Geometry: final body of the model. Coordinates: model frame, mm. Face numbers are marked on the shaded views. A direction names the side the tool comes from. Give positions to 0.01 mm unless a question says otherwise; leave off trailing zeros. Write each loop counter-clockwise with the first axis right and the second up, starting at its lowest first coordinate (ties: lowest second). Pieces come first, ordered by that corner, then holes. Notation, with made-up numbers: (62, 38.5) -> (101, 38.5) arc R22 cw to (101, 54.5) -> close; hole circle Ø10 at (77.5, -15.75). An arc over 180 degrees is marked (long way). Answer in a Markdown table with one row per item. Add a question column.
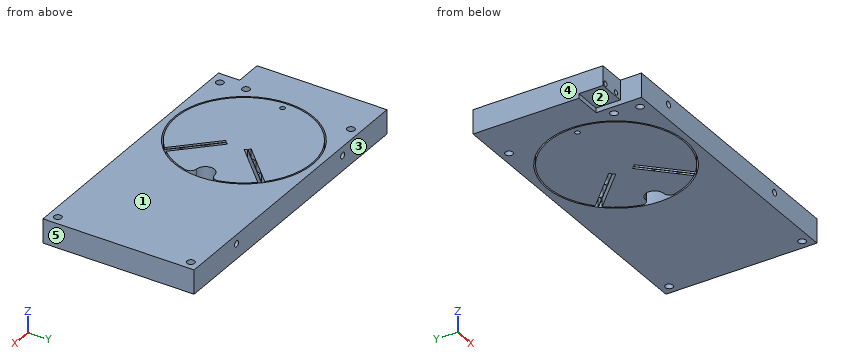
Autodesk Inventor part; units mm, degrees
ref_plane "YZ Plane" through (0, 0, 0) normal (1, 0, 0) x (0, 1, 0)
ref_plane "XZ Plane" through (0, 0, 0) normal (0, 1, 0) x (-1, 0, 0)
ref_plane "XY Plane" through (0, 0, 0) normal (0, 0, 1) x (1, 0, 0)
sketch "Sketch1" plane through (0, 0, 0) normal (0, 0, 1) x (1, 0, 0)
  line L0 (0, 0) -> (100, 0)
  line L1 (100, 0) -> (100, 50)
  line L2 (100, 50) -> (0, 50)
  line L3 (0, 50) -> (0, 0)
  circle A0 centre (95, 45) radius 1.75
  circle A1 centre (95, 5) radius 1.75
  circle A2 centre (15, 45) radius 1.75
  circle A3 centre (15, 5) radius 1.75
  dimension "d0" = 50
  dimension "d1" = 100
  dimension "d2" = 5
  dimension "d3" = 5
  dimension "d4" = 5
  dimension "d5" = 5
  dimension "d6" = 5
  dimension "d7" = 15
  dimension "d8" = 15
  dimension "d9" = 5
  dimension "d10" = 3.5
  dimension "d11" = 3.5
  dimension "d12" = 3.5
  dimension "d13" = 3.5
extrude "Extrusion1" add sketch "Sketch1" along normal blind 8 contours L3 L2 L1 L0 | A0 | A1 | A2 | A3
sketch "Sketch4" plane through (0, 0, 8) normal (0, 0, 1) x (1, 0, 0)
  circle A0 centre (15, 25) radius 0.8
  circle A1 centre (55, 25) radius 3
  line L0 (0, 50) -> (0, 0)
  line L1 (35, 25) -> (52.9141, 42.9141)
  line L2 (35, 25) -> (41.4896, 25)
  line L3 (35, 25) -> (55.1987, 4.8013)
  circle A2 centre (35, 25) radius 23
  line L4 (0, 0) -> (100, 0)
  circle A3 centre (35, 25) radius 5
  line L5 (38.5, 28.5707) -> (51.2281, 41.2988)
  line L6 (37.757, 29.1712) -> (50.1871, 41.6013)
  line L7 (38.5707, 28.5) -> (51.2988, 41.2281)
  line L8 (51.6013, 40.1871) -> (39.1712, 27.757)
  line L9 (38.5707, 21.5) -> (51.2988, 8.7719)
  line L10 (38.5, 21.4293) -> (51.2281, 8.7012)
  line L11 (37.757, 20.8288) -> (50.1871, 8.3987)
  line L12 (39.1712, 22.243) -> (51.6013, 9.8129)
  arc A4 (51.6013, 9.8129) -> (50.1871, 8.3987) centre (35, 25) ccw
  circle A5 centre (41.2925, 32.7067) radius 0.95
  circle A6 centre (42.7067, 34.121) radius 0.95
  circle A7 centre (46.2423, 37.6565) radius 0.95
  circle A8 centre (47.6565, 39.0707) radius 0.95
  circle A9 centre (42.7067, 18.7075) radius 0.95
  circle A10 centre (44.121, 17.2933) radius 0.95
  circle A11 centre (47.6565, 13.7577) radius 0.95
  circle A12 centre (49.0707, 12.3435) radius 0.95
  point P0 (0, 15)
  point P1 (7, 0)
  point P2 (57.4312, 26.7576)
  point P3 (57.4312, 23.2424)
  point P4 (58, 25)
  point P5 (50.9452, 40.8745)
  point P6 (50.8745, 40.9452)
  point P7 (41.9643, 32.035)
  point P8 (41.9643, 33.3785)
  point P9 (42.035, 33.4492)
  point P10 (43.3785, 33.4492)
  point P11 (46.914, 36.9847)
  point P12 (46.914, 38.3282)
  point P13 (48.3282, 38.399)
  point P14 (46.9847, 38.399)
  point P15 (42.035, 18.0357)
  point P16 (43.3785, 18.0357)
  point P17 (43.4492, 17.965)
  point P18 (43.4492, 16.6215)
  point P19 (46.9847, 13.086)
  point P20 (48.3282, 13.086)
  point P21 (48.399, 13.0153)
  point P22 (48.399, 11.6718)
  dimension "d34" = 10
  dimension "d22" = 15
  dimension "d23" = 40
  dimension "d24" = 20
  dimension "d26" = 1.6
  dimension "d27" = 6
  dimension "d28" = 45
  dimension "d29" = 45
  dimension "d30" = 46
  dimension "d31" = 25
  dimension "d32" = 25
  dimension "d33" = 25
  dimension "d35" = 1
  dimension "d36" = 1
  dimension "d37" = 0.1
  dimension "d38" = 0.05
  dimension "d39" = 0.1
  dimension "d40" = 0.05
  dimension "d41" = 1
  dimension "d42" = 1
  dimension "d79" = 5
  dimension "d80" = 2
  dimension "d81" = 5
  dimension "d82" = 2
  dimension "d83" = 5
  dimension "d84" = 2
  dimension "d85" = 5
  dimension "d86" = 2
extrude "Extrusion4" cut sketch "Sketch4" against normal blind 8 contours A0 | A1 A4 | A2 L9 A12 L12 A4 A1 | A1 A4 L7 A2 | A4 A1 | L8 A3 L7 A4 | A12 L12 | L5 A4 L11 A3 L10 A2 | L9 A10 L12 A11 | A11 L12 | L5 A8 L6 A4 | A3 L12 A9 L9 | A10 L12 | A3 L6 A5 L5 | A8 L6 | A9 L12 | A5 L6 | L5 A6 L6 A7 | A7 L6 | A6 L6 picked at (49.0352, 12.0288) picked at (47.3576, 13.4145) picked at (44.1564, 16.9786) picked at (47.9671, 39.0089) picked at (42.6021, 18.4086) picked at (41.6092, 32.7067) picked at (46.2068, 37.3418) picked at (43.0173, 33.7349)
fillet "Fillet2" radius 2 2 edges at (57.4312, 26.7576, 4) (57.4312, 23.2424, 4)
sketch "Sketch5" plane through (0, 0, 0) normal (-1, 0, 0) x (0, 0, 1)
  line L0 (0, 0) -> (1.5, 0)
  line L1 (1.5, 0) -> (1.5, 15)
  line L2 (1.5, 15) -> (0, 15)
  line L3 (0, 15) -> (0, 0)
  line L4 (8, 0) -> (8, 50)
  line L5 (8, 0) -> (1.5, 0)
  line L6 (1.5, 0) -> (1.5, 7)
  line L7 (1.5, 7) -> (8, 7)
  line L8 (8, 7) -> (8, 0)
  dimension "d47" = 15
  dimension "d48" = 1.5
  dimension "d51" = 7
extrude "Extrusion5" cut sketch "Sketch5" against normal blind 9
sketch "Sketch6" plane through (0, 7, 1.5) normal (0, -1, 0) x (1, 0, 0)
  circle A0 centre (6.75, 1.2764) radius 1.1
  circle A1 centre (1.25, 1.2764) radius 1.1
  circle A2 centre (6.75, 1.2764) radius 0.8
  circle A3 centre (1.25, 1.2764) radius 0.8
  point P0 (0, -1.5)
  dimension "d52" = 1.6
  dimension "d53" = 1.6
extrude "Extrusion6" cut sketch "Sketch6" against normal blind 8 contours A2 | A3
sketch "Sketch7" plane through (0, 0, 8) normal (0, 0, 1) x (1, 0, 0)
  circle A0 centre (97, 3) radius 1.7
  circle A1 centre (97, 47) radius 1.7
  circle A2 centre (12, 11) radius 1.7
  circle A3 centre (21.5, 47.5) radius 1.7
  circle A4 centre (97, 3) radius 1.25
  circle A5 centre (97, 47) radius 1.25
  circle A6 centre (13, 3) radius 1.25
  circle A7 centre (12, 11) radius 1.25
  circle A8 centre (21.5, 47.5) radius 1.25
  circle A9 centre (14, 47) radius 1.7
  circle A10 centre (14, 47) radius 1.25
  line L0 (9, 0) -> (100, 0)
  line L1 (9, 0) -> (9, 15)
  point P0 (0, 0)
  dimension "d56" = 2.5
  dimension "d57" = 2.5
  dimension "d58" = 2.5
  dimension "d59" = 2.5
  dimension "d60" = 2.5
  dimension "d63" = 2.5
  dimension "d64" = 3
  dimension "d65" = 4
extrude "Extrusion7" cut sketch "Sketch7" against normal blind 8 contours A4 | A5 | A6 | A7 | A10
sketch "Sketch8" plane through (0, 50, 0) normal (0, 1, 0) x (1, 0, 0)
  circle A0 centre (23, -5) radius 1.375
  circle A1 centre (78, -5) radius 1.375
  circle A2 centre (23, -5) radius 1.025
  circle A3 centre (78, -5) radius 1.025
  line L0 (0, 0) -> (0, -8)
  dimension "d68" = 2.05
  dimension "d69" = 2.05
  dimension "d74" = 23
  dimension "d75" = 23
  dimension "d76" = 55
extrude "Extrusion8" cut sketch "Sketch8" against normal blind 8 contours A2 | A3
sketch "Sketch9" plane through (100, 0, 0) normal (0, -1, 0) x (1, 0, 0)
  circle A0 centre (-77, 5) radius 1.375
  circle A1 centre (-22, 5) radius 1.375
  circle A2 centre (-77, 5) radius 1.025
  circle A3 centre (-22, 5) radius 1.025
  line L0 (-100, 1.5) -> (-100, 8)
  point P0 (-100, 0)
  dimension "d70" = 2.05
  dimension "d71" = 2.05
  dimension "d77" = 23
  dimension "d78" = 55
extrude "Extrusion9" cut sketch "Sketch9" against normal blind 8 contours A2 | A3
equation "\"d4\" = d3"
equation "\"d5\" = d2"
equation "\"d6\" = d3"
equation "\"d9\" = d4"
equation "\"d10\" = d11"
equation "\"d12\" = d11"
equation "\"d13\" = d11"
equation "\"d24\" = 0.5 * d23"
equation "\"d37\" = BladeThicknessRCC"
equation "\"d38\" = 0.5 * d37"
equation "\"d39\" = BladeThicknessRCC"
equation "\"d40\" = 0.5 * BladeThicknessRCC"
equation "\"d59\" = d58"
equation "\"d60\" = d59"
equation "\"d75\" = d74"
equation "\"bladeThicknessTablePushing\" = 0.1"
equation "\"bladeThicknessTable\" = 0.1"
equation "\"bladeThicknessForceConverter\" = 0.2"
equation "\"bladeThicknessWheelAnchor\" = 0.1"
equation "\"safetyPlay\" = 0.1"
equation "\"OffsetMotorSpring\" = -1"
equation "\"BladeThicknessRCC\" = 0.1"
equation "\"bladeThicknessZeroConverter\" = 0.1"
equation "\"rangeXProbeMin\" = -0.6"
equation "\"thicknessWheelPlate\" = 8"
equation "\"rangeXProbeMax\" = 0.6"
equation "\"BladeLengthRCC\" = 18"
equation "\"bladeLengthTable\" = 18"
equation "\"bladeLengthWheelAnchor\" = 7.5"
equation "\"RCCdeadCenter\" = 5"
equation "\"bladeLengthZeroConverter\" = 11.98"
equation "\"bladeLengthTablePushing\" = 12"
equation "\"bladeLengthForceConverter\" = 12.125"
equation "\"thicknessConverterPlate\" = 4"
properties part number "RoueV3partA"
Q1. Section B-B on x = 46. Return loops of the section in (y, z), and give its area (3 significant figures).
Q2. Pull-direction query (X, two-part tool) for the marked faces 3, 4 and 5; classes: +X half, -X half, draft (parallel to the pull), parting line (faces both ways), or undercut.
Q3. Contact query for flat-ended pins moving along their axis: pin 1 Ø2.5 at (x, z) = (23, 5) entering from -Y; pin 2 Ø1.3 at (x, z) = (6.5, 2.5) entering from -Y; pin 3 Ø1.8 at (x, z) = (78, 5) entering from -Y; pin 4 Ø4 at (x, y) = (6, 12) entering from -Z. Output: stop coordinate, or through.
Q4. Line query: probe 1 along Z at (x, y) = (78, 44) (3 decimals); probe 2 along X at (y, z) = (23.5, 6.25); probe 3 along X at (y, z) = (12, 7). Output: solid intervals per line, ascending. Write a range as from..to.
Q5. Access query for the marked faces 1 and 2. Directions: +Z, -Z, +X, -X, +Y, -Y. A direction counts if a zero-diameter tool reaches every point of the face in a straight line with its end or side. Return the directions, or none.
Q6. Section A-A on x = 35. Return loops of the section in (y, z), and give its area (3 significant figures).
Checks:
| question | item | result |
|---|---|---|
| 1 | outline | (0, 0) -> (4.8, 0) -> (4.8, 8) -> (0, 8) -> close; (5.37, 0) -> (12.59, 0) -> (12.59, 8) -> (5.37, 8) -> close; (13.93, 0) -> (14.07, 0) -> (14.07, 8) -> (13.93, 8) -> close; (15.41, 0) -> (34.59, 0) -> (34.59, 8) -> (15.41, 8) -> close; (35.93, 0) -> (36.07, 0) -> (36.07, 8) -> (35.93, 8) -> close; (37.41, 0) -> (44.63, 0) -> (44.63, 8) -> (37.41, 8) -> close; (45.2, 0) -> (50, 0) -> (50, 8) -> (45.2, 8) -> close |
| 1 | area | 348 mm^2 |
| 2 | face 3 | draft |
| 2 | face 4 | -X half |
| 2 | face 5 | +X half |
| 3 | pin 1 | y = 0 |
| 3 | pin 2 | y = 7 |
| 3 | pin 3 | y = 8 |
| 3 | pin 4 | z = 1.5 |
| 4 | probe 1 | 0..3.975, 6.025..8 |
| 4 | probe 2 | 0..12.05, 12.55..52.4, 57.95..100 |
| 4 | probe 3 | 0..11.25, 12.75..16.03, 16.64..46.59, 47.93..48.18, 49.41..53.36, 53.97..100 |
| 5 | face 1 | +Z, +X, -X, +Y, -Y |
| 5 | face 2 | -Z, -X, -Y |
| 6 | outline | (0, 0) -> (2, 0) -> (2, 8) -> (0, 8) -> close; (2.5, 0) -> (47.5, 0) -> (47.5, 8) -> (2.5, 8) -> close; (48, 0) -> (50, 0) -> (50, 8) -> (48, 8) -> close |
| 6 | area | 392 mm^2 |
